Part print with two shaded views. Sizes in mm from the minimum x, y, z corner. A direction names the side the tool comes from. Coordinates: 2 decimals unless noted, no trailing zeros. Order: outer loops, then holes, each group sorted by start corner. A loop starts at its lowest first (then second) coordinate and runs counter-clockwise, first axis right, second up. Notation, with made-up numbers: (60.5, 39) - (112.5, 39) arc R14 cw to (112.5, 59) - close; hole circle Ø6 at (68.25, -34). An arc over 180 degrees is marked (long way). One line per item, written item: value.
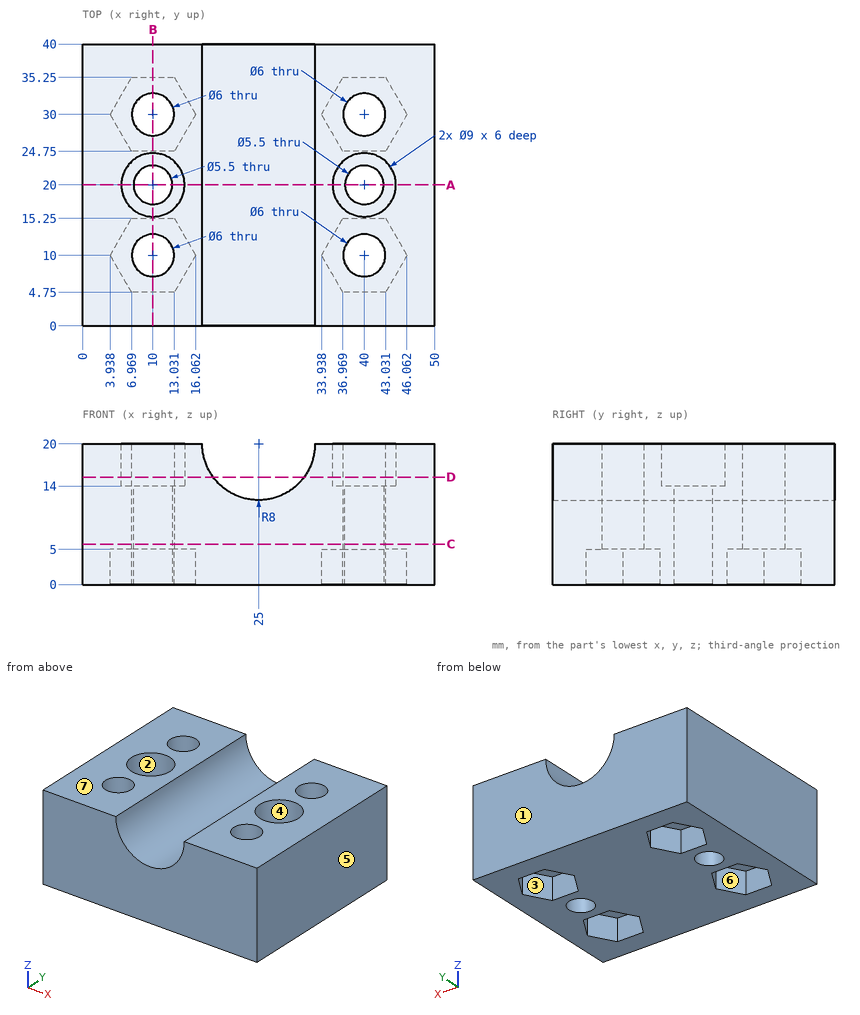
1. Probe line 1 along Y through (x, z) = (10, 7); line 2 along Y through (x, z) = (10, 18.85); line 3 along X through (y, z) = (5, 13.75) (1 decimal). List the from-to ranges inside material, lowest first.
Values found:
line 1: y = 0 to 7, 13 to 17.25, 22.75 to 27, 33 to 40
line 2: y = 0 to 7, 13 to 15.5, 24.5 to 27, 33 to 40
line 3: x = 0 to 20, 30 to 50
2. Band-saw the part on B-B, the plane x = 10. Give the cut face in (y, z), and give its area (3 significant figures).
Values found:
outline: (0, 0) - (4.75, 0) - (4.75, 5) - (7, 5) - (7, 20) - (0, 20) - close; (13, 5) - (15.25, 5) - (15.25, 0) - (17.25, 0) - (17.25, 14) - (15.5, 14) - (15.5, 20) - (13, 20) - close; (22.75, 0) - (24.75, 0) - (24.75, 5) - (27, 5) - (27, 20) - (24.5, 20) - (24.5, 14) - (22.75, 14) - close; (33, 5) - (35.25, 5) - (35.25, 0) - (40, 0) - (40, 20) - (33, 20) - close
area: 384 mm2
3. Two-plate mould, pull along X, no slides. Class the marked faces 4, 5, 6 and 7: pulls with the +X half, pulls with the -X half, needs draft (parallel to the pull), parting line crosses it, or undercut.
Values found:
face 4: undercut
face 5: pulls with the +X half
face 6: undercut
face 7: needs draft
4. Flat gauge pins, fed straight in: P1, Ø8.5, axis at x = 41, y = 9, coming from the -Z side; P2, Ø5, axis at x = 41.5, y = 31, coming from the -Z side. Where does each tip first touch, or does it go through?
Values found:
P1: stops at z = 0
P2: stops at z = 5
5. Band-saw the part on C-C, the plane z = 5.75. Give the cut face in (x, y), and give its area (3 significant figures).
Values found:
outline: (0, 0) - (50, 0) - (50, 40) - (0, 40) - close; hole circle Ø6 at (10, 10); hole circle Ø6 at (10, 30); hole circle Ø5.5 at (10, 20); hole circle Ø6 at (40, 10); hole circle Ø6 at (40, 30); hole circle Ø5.5 at (40, 20)
area: 1,840 mm2
6. 3-axis set-ups, long thin cutter, end or side, ignore diameter. For the marked faces 1, 2 and 3: which of +Z, -Z, +X, -X, +Y, -Y reach the whole face in a straight line?
Values found:
face 1: +Z, -Z, +X, -X, +Y
face 2: +Z
face 3: -Z
7. Band-saw the part on D-D, the plane z = 15.25. Give the cut face in (x, y), and give its area (3 significant figures).
Values found:
outline: (0, 0) - (18.56, 0) - (18.56, 40) - (0, 40) - close; (31.44, 0) - (50, 0) - (50, 40) - (31.44, 40) - close; hole circle Ø9 at (10, 20); hole circle Ø6 at (10, 10); hole circle Ø6 at (10, 30); hole circle Ø9 at (40, 20); hole circle Ø6 at (40, 10); hole circle Ø6 at (40, 30)
area: 1,240 mm2
8. Band-saw the part on A-A, the plane y = 20. Give the cut face in (x, z).
Values found:
outline: (0, 0) - (7.25, 0) - (7.25, 14) - (5.5, 14) - (5.5, 20) - (0, 20) - close; (12.75, 0) - (37.25, 0) - (37.25, 14) - (35.5, 14) - (35.5, 20) - (33, 20) arc R8 cw to (17, 20) - (14.5, 20) - (14.5, 14) - (12.75, 14) - close; (42.75, 0) - (50, 0) - (50, 20) - (44.5, 20) - (44.5, 14) - (42.75, 14) - close
